Here's the drawing with two shaded views (mm, measured from the low corner). I have some questions. A direction names the side the tool comes from. Give positions to 0.01 mm unless a question says otherwise; leave off trailing zeros. Loops run counter-clockwise (first coordinate to the right, second up) from the corner with the lowest first, then second, coordinate; pieces in that order, holes last. Notation, with made-up numbers: (64, -11.75) - (76, -11.75) arc R21 ccw to (76, 5.25) - close; hole circle Ø9 at (60, 63). An arc over 180 degrees is marked (long way). Use a Markdown table: item, result. Add a question column.
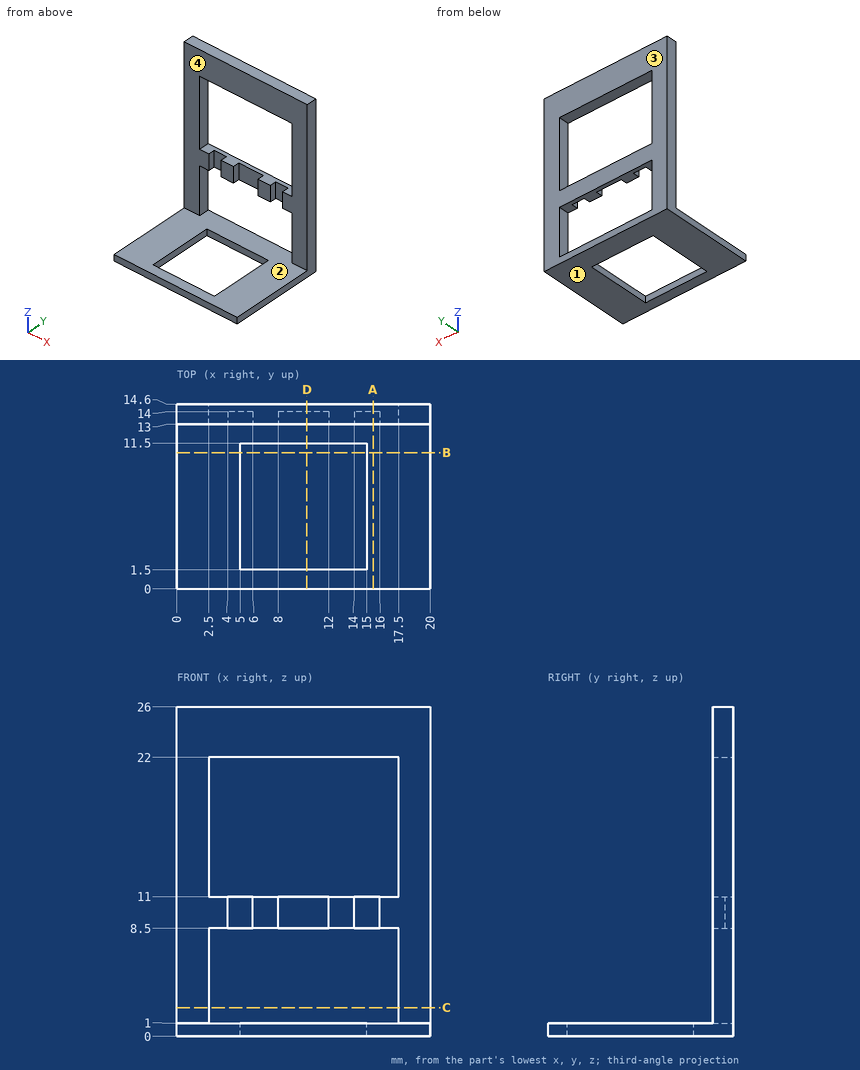
1. Will these pins go through, and if not, where does the flat tip stop? P1, Ø0.6, axis at x = 13, z = 9.5, coming from the -Y side; P2, Ø1, axis at x = 15, z = 9.5, coming from the -Y side.
2. Suppose I cut it at B-B (y = 10.75). List the corners of the cut face in (x, z) for me.
3. If we mould it in two halves opening along X, with no side actions, what happens to the marked faces 1 and 2? For each: released by +X, released by -X, zero draft, split by the parting line, or undercut.
4. On a 3-axis mill with a long thin cutter (end or side, diameter ignored), from which of +Z, -Z, +X, -X, +Y, -Y can I reach the whole of each face in a straight line? I mean the marked faces 3 and 4. Say none if no direction works.
5. Please list where these lines run through material, in increasing order: line 1 along Z through (x, y) = (10.25, 13.5); line 2 along Z through (x, y) = (1.25, 3.5); line 3 along Y through (x, z) = (5.75, 10.5). Write a range as [from, to].
6. Suppose I cut it at A-A (x = 15.5). List the corners of the cut face in (y, z) for me.
7. Suppose I cut it at C-C (z = 2.25). List the corners of the cut face in (x, y) for me.
8. Suppose I cut it at D-D (x = 10.25). List the corners of the cut face in (y, z) for me.
Results below:
| question | item | result |
|---|---|---|
| 1 | P1 | y = 13 |
| 1 | P2 | y = 14 |
| 2 | outline | (0, 0) - (5, 0) - (5, 1) - (0, 1) - close; (15, 0) - (20, 0) - (20, 1) - (15, 1) - close |
| 3 | face 1 | zero draft |
| 3 | face 2 | undercut |
| 4 | face 3 | +Z, -Z, +X, -X, +Y |
| 4 | face 4 | +Z, +X, -X, -Y |
| 5 | line 1 | [0, 1], [22, 26] |
| 5 | line 2 | [0, 1] |
| 5 | line 3 | [14, 14.6] |
| 6 | outline | (0, 0) - (14.6, 0) - (14.6, 1) - (0, 1) - close; (13, 22) - (14.6, 22) - (14.6, 26) - (13, 26) - close; (14, 8.5) - (14.6, 8.5) - (14.6, 11) - (14, 11) - close |
| 7 | outline | (0, 13) - (2.5, 13) - (2.5, 14.6) - (0, 14.6) - close; (17.5, 13) - (20, 13) - (20, 14.6) - (17.5, 14.6) - close |
| 8 | outline | (0, 0) - (1.5, 0) - (1.5, 1) - (0, 1) - close; (11.5, 0) - (14.6, 0) - (14.6, 1) - (11.5, 1) - close; (13, 22) - (14.6, 22) - (14.6, 26) - (13, 26) - close; (14, 8.5) - (14.6, 8.5) - (14.6, 11) - (14, 11) - close |
